```python
from build123d import *

# Parameters (mm, degrees)
SKETCH1_W           = 30
SKETCH1_H           = 30
BOSS_EXTRUDE1_DEPTH = 10
SKETCH3_R           = 2
BOSS_EXTRUDE4_DEPTH = 50
SKETCH4_W           = 30
SKETCH4_H           = 30
BOSS_EXTRUDE5_DEPTH = 5
CAVITY1_START       = 12.5
CAVITY1_OUTLINE_W   = 5
CAVITY1_OUTLINE_H   = 10
CAVITY1_DEPTH       = 5


# Read off the part's stored shape, not the designer's step: Cavity1
with BuildPart() as part:
    # Sketch1 → Boss-Extrude1 (new body)
    with BuildSketch(Plane.XY):
        with Locations((15, 15)):
            Rectangle(SKETCH1_W, SKETCH1_H)
    extrude(amount=BOSS_EXTRUDE1_DEPTH)

    # Sketch3 → Boss-Extrude4 (add)
    with BuildSketch(Plane(origin=(0, 0, 0), x_dir=(-1, 0, 0), z_dir=(0, 0, -1))):
        with Locations((-27, 3)):
            Circle(SKETCH3_R)
    extrude(amount=BOSS_EXTRUDE4_DEPTH)

    # Sketch4 → Boss-Extrude5 (add)
    with BuildSketch(Plane(origin=(0, 0, -50), x_dir=(-1, 0, 0), z_dir=(0, 0, -1))):
        with Locations((-15, 15)):
            Rectangle(SKETCH4_W, SKETCH4_H)
    extrude(amount=BOSS_EXTRUDE5_DEPTH)

    # Cavity1 outline → Cavity1 (cut)
    with BuildSketch(Plane.YZ.offset(CAVITY1_START)):
        with Locations((15, 5)):
            Rectangle(CAVITY1_OUTLINE_W, CAVITY1_OUTLINE_H)
    extrude(amount=CAVITY1_DEPTH, mode=Mode.SUBTRACT)


solid = part.part
```
Verification items for the finished model (mm, model axes). A direction names the side the tool comes from. Give positions to 0.01 mm unless a question says otherwise; leave off trailing zeros. Order: outer loops, then holes, each group sorted by start corner. A loop starts at its lowest first (then second) coordinate and runs counter-clockwise, first axis right, second up. Notation, with made-up numbers: (35, 89.25) -> (52, 89.25) arc R23 cw to (52, 121.25) -> close; hole circle Ø10 at (-21, -26). An arc over 180 degrees is marked (long way). One line per item, written item: value.
(1) Sectioned sample at A-A on x = 19.5. Record the cut outline in (y, z).
Final values:
outline: (0, -55) -> (30, -55) -> (30, -50) -> (0, -50) -> close; (0, 0) -> (30, 0) -> (30, 10) -> (0, 10) -> close
(2) Tool access check on faces 4 (the face through (25.092, 3.601, -24.65)), 5 (the face through (15, 30, 5)), 6 (the face through (15, 17.5, 5)). Record the directions out of +Z, -Z, +X, -X, +Y, -Y that give a thin tool (end or side, any length) a straight path to the whole face; none if there is none.
Final values:
face 4: none
face 5: +Z, -Z, +X, -X, +Y
face 6: +Z
(3) Sectioned sample at C-C on z = 4. Record the cut outline in (x, y), then the cut area to 3 significant figures.
Final values:
outline: (0, 0) -> (30, 0) -> (30, 30) -> (0, 30) -> close; hole (12.5, 12.5) -> (17.5, 12.5) -> (17.5, 17.5) -> (12.5, 17.5) -> close
area: 875 mm^2
(4) Scan lines: line 1 along Z through (x, y) = (10.75, 17.75); line 2 along X through (y, z) = (15, 1). Record each from-to range of solid material in increasing order. Write a range as [from, to].
Final values:
line 1: [-55, -50], [0, 10]
line 2: [0, 12.5], [17.5, 30]
(5) Draft check along Y on faces 1 (the face through (11, 15, 0)), 2 (the face through (15, 12.5, 5)), 3 (the face through (15, 0, -52)). Enter one of: pulls with the +Y half, pulls with the -Y half, needs draft (parallel to the pull), parting line crosses it, or undercut.
Final values:
face 1: needs draft
face 2: undercut
face 3: pulls with the -Y half
(6) Sectioned sample at D-D on y = 3. Record the cut outline in (x, z), then the cut area to 3 significant figures.
Final values:
outline: (0, -55) -> (30, -55) -> (30, -50) -> (29, -50) -> (29, 0) -> (30, 0) -> (30, 10) -> (0, 10) -> (0, 0) -> (25, 0) -> (25, -50) -> (0, -50) -> close
area: 650 mm^2
